Check sheet for the modelled part. Datum: model origin and axes. Units: mm. Round coordinates to 2 decimals unless told otherwise and drop trailing zeros. Order: outer loops, then holes, each group sorted by start corner. A loop starts at its lowest first (then second) coordinate and runs counter-clockwise, first axis right, second up. Notation, with made-up numbers: M -33,86 L 21,86 A21 cw 21,124 Z; hole C 25.25,7.25 d1. An arc over 180 degrees is marked long. One line per item, written item: value. Start each with the question number.
(1) Cross-section at B-B, the plane y = -22. Enter the section's corners in (x, z).
(2) Depth check by flat-ended pin: pin 1 Ø5.5 at (y, z) = (0, 23.81) entering from -X; pin 2 Ø1 at (x, y) = (-7.5, 29) entering from -Z; pin 3 Ø2 at (x, y) = (5.5, -8.5) entering from +Z. Enter the tip coordinate at first touch or a pass-through.
(3) Thickness scan on L1, parallel to Z at x = 3, y = -11.5; L2, parallel to Z at x = 13, y = 26. Record the ranges inside material, lowest first.
from build123d import *

# Parameters (mm, degrees)
SKETCH1_W                       = 38.1
SKETCH1_H                       = 88.9
BOSS_EXTRUDE1_DEPTH             = 1143
F_9_32_0_28125_DIAMETER_HOLE1_D = 7.14375
SKETCH5_R                       = 3.571875
CUT_EXTRUDE1_DEPTH              = 39.1


with BuildPart() as part:
    # Sketch1 → Boss-Extrude1 (new body)
    with BuildSketch(Plane.XY):
        Rectangle(SKETCH1_W, SKETCH1_H)
    extrude(amount=BOSS_EXTRUDE1_DEPTH)

    # 9/32 (0.28125) Diameter Hole1 (through all)
    with Locations(Plane(origin=(19.05, 0, 0), x_dir=(0, 0, -1), z_dir=(1, 0, 0))):
        with Locations((-1128.7125, 0), (-23.8125, 0)):
            Hole(F_9_32_0_28125_DIAMETER_HOLE1_D / 2)

    # Sketch5 → Cut-Extrude1 (cut, through all)
    with BuildSketch(Plane(origin=(19.05, 0, 0), x_dir=(0, 0, -1), z_dir=(1, 0, 0))):
        Polygon((-866.812642201, -44.45), (-993.775, 44.45), (-1143, 44.45), (-1143, -44.45), (-869.95, -44.45), align=None)
        with Locations((-1128.7125, 0)):
            Circle(SKETCH5_R, mode=Mode.SUBTRACT)
    extrude(amount=-CUT_EXTRUDE1_DEPTH, mode=Mode.SUBTRACT)


solid = part.part
Values found:
1. outline: M -19.05,0 L 19.05,0 L 19.05,898.87 L -19.05,898.87 Z
2. pin 1: through
2. pin 2: z = 0
2. pin 3: z = 919.58
3. L1: 0 to 913.87
3. L2: 0 to 967.43
